Source: three-view drawing plus pictorial views. Frame: mm from the lowest corner of the part. A direction names the side the tool comes from. Give positions to 0.01 mm unless a question says otherwise; leave off trailing zeros. Loops run counter-clockwise (first coordinate to the right, second up) from the corner with the lowest first, then second, coordinate; pieces in that order, holes last. Notation, with made-up numbers: (-20.75, 40.25) -> (37.25, 40.25) arc R21 cw to (37.25, 54.25) -> close; hole circle Ø9 at (12, 20.25). An arc over 180 degrees is marked (long way). One line per item, written item: value. Start each with the question number.
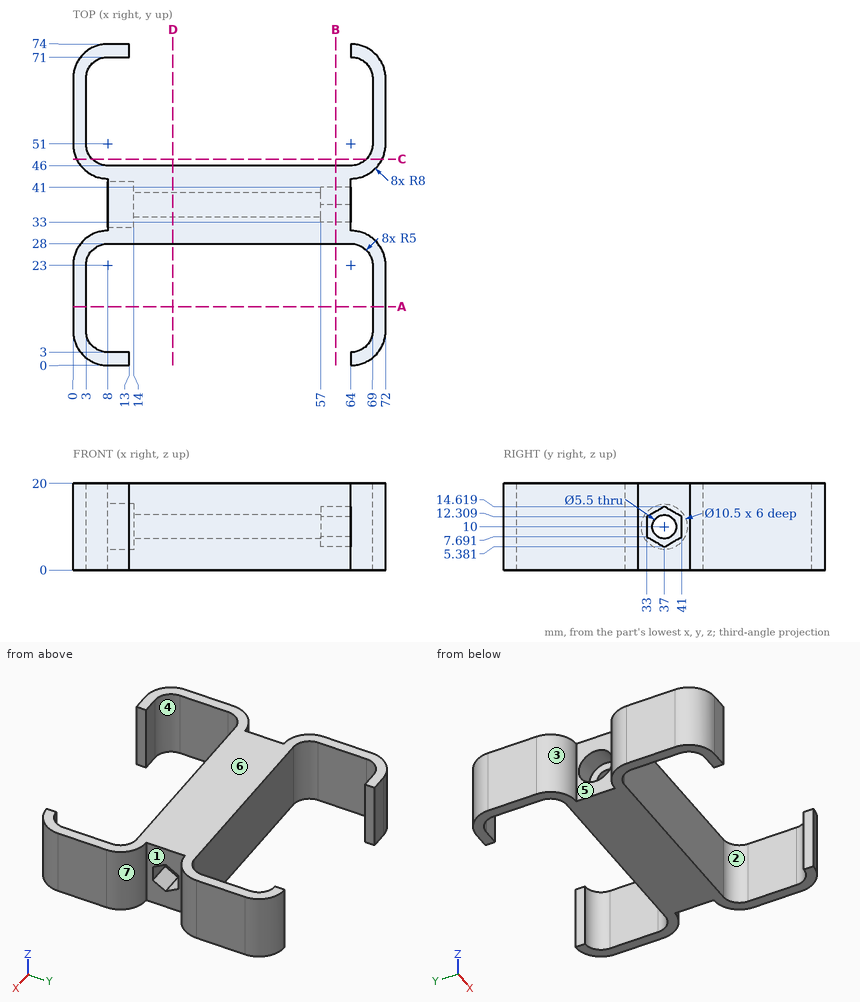
Item 1: Section B-B, the plane x = 60.5. Output: boundary loops of the cut face in (y, z).
Item 2: Section C-C, the plane y = 47.5. Output: boundary loops of the cut face in (x, z), then the cut area to 3 significant figures.
Item 3: Section A-A, the plane y = 13.5. Output: boundary loops of the cut face in (x, z), then the cut area to 3 significant figures.
Item 4: Section D-D, the plane x = 23. Output: boundary loops of the cut face in (y, z), then the cut area to 3 significant figures.
Item 5: Ray query, line 1 along X through (y, z) = (64, 12.5); line 2 along Y through (x, z) = (66.5, 9.75); line 3 along Y through (x, z) = (12, 6.75) (1 decimal). Return the intervals inside material, ascending. Write a range as [from, to].
Item 6: Access query for the marked faces 1, 2 and 3. Directions: +Z, -Z, +X, -X, +Y, -Y. A direction counts if a zero-diameter tool reaches every point of the face in a straight line with its end or side. Return the directions, or none.
Item 7: Mould query, pull axis X, two halves, no side actions, for the marked faces 4, 5, 6 and 7. Classes: pulls with the +X half, pulls with the -X half, needs draft (parallel to the pull), parting line crosses it, or undercut.
Item 8: Pin query (flat end, axial travel): pin 1 (0.9 mm diameter, centred on y = 1, z = 11, fed in from +X) (1 decimal); pin 2 (6 mm diameter, centred on x = 26, z = 4, fed in from -Y); pin 3 (8.5 mm diameter, centred on y = 37, z = 10, fed in from +X). Return the tip coordinate at first contact, or that it passes through.
Geometry check:
1. outline: (28, 0) -> (46, 0) -> (46, 20) -> (28, 20) -> close; hole (33, 7.69) -> (37, 5.38) -> (41, 7.69) -> (41, 12.31) -> (37, 14.62) -> (33, 12.31) -> close
2. outline: (0.81, 0) -> (4.43, 0) -> (4.43, 20) -> (0.81, 20) -> close; (67.57, 0) -> (71.19, 0) -> (71.19, 20) -> (67.57, 20) -> close
2. area: 145 mm2
3. outline: (0, 0) -> (3, 0) -> (3, 20) -> (0, 20) -> close; (69, 0) -> (72, 0) -> (72, 20) -> (69, 20) -> close
3. area: 120 mm2
4. outline: (28, 0) -> (46, 0) -> (46, 20) -> (28, 20) -> close; hole circle Ø5.5 at (37, 10)
4. area: 336 mm2
5. line 1: x = [0, 3], [69, 72]
5. line 2: y = [0.4, 3.67], [27.33, 30.6], [43.4, 46.67], [70.33, 73.6]
5. line 3: y = [0, 3], [28, 32.9], [41.1, 46], [71, 74]
6. face 1: +Z, -Z, +X
6. face 2: +Z, -Z
6. face 3: +Z, -Z, -X
7. face 4: undercut
7. face 5: pulls with the -X half
7. face 6: needs draft
7. face 7: pulls with the +X half
8. pin 1: stops at x = 68.6
8. pin 2: stops at y = 28
8. pin 3: stops at x = 64
